from build123d import *

# Parameters (mm, degrees)
SKETCH_1_R          = 3
EXTRUDE_1_DEPTH     = 15
SKETCH_2_R          = 5
CUT_EXTRUDE_1_DEPTH = 30


with BuildPart() as part:
    # 草图1 → 凸台-拉伸1 (new, symmetric)
    with BuildSketch(Plane.XY):
        with BuildLine():
            Line((8, 0), (12, 0))
            ThreePointArc((12, 0), (17.656854249, -2.343145751), (20, -8))
            Line((20, -8), (20, -180))
            Line((20, -180), (0, -180))
            Line((0, -180), (0, -8))
            ThreePointArc((0, -8), (2.343145751, -2.343145751), (8, 0))
        make_face()
        with Locations((8, -8)):
            Circle(SKETCH_1_R, mode=Mode.SUBTRACT)
    extrude(amount=EXTRUDE_1_DEPTH, both=True)

    # 草图2 → 切除-拉伸1 (cut)
    with BuildSketch(Plane.XZ.offset(180)):
        with Locations(Location((10, 0, 0), (0, 0, 270))):
            Circle(SKETCH_2_R)
    extrude(amount=-CUT_EXTRUDE_1_DEPTH, mode=Mode.SUBTRACT)


solid = part.part
Model file for the job. Use its own axes, mm. A direction names the side the tool comes from. Round coordinates to 2 decimals unless told otherwise and drop trailing zeros. Loops run counter-clockwise (first coordinate to the right, second up) from the corner with the lowest first, then second, coordinate; pieces in that order, holes last.
1. Wall check: probe 1 along X at (y, z) = (-169.5, 0); probe 2 along Y at (x, z) = (8, -2.5); probe 3 along Y at (x, z) = (8, -4.75). Give the ranges that are in metal, low to high.
Check values:
probe 1: x = 0 to 5, 15 to 20
probe 2: y = -150 to -11, -5 to 0
probe 3: y = -180 to -11, -5 to 0
2. Tool access for faces 4 (the cylindrical face through (17.594, -2.281, 0.21)), 5 (the cylindrical face through (14.957, -165.21, 0.651)): list every direction of +Z, -Z, +X, -X, +Y, -Y with a clear straight run to the whole face (end or side of a thin tool).
Check values:
face 4: +Z, -Z, +X, +Y
face 5: -Y
3. Mould opens along X. For faces 1 (the flat face through (10, -150, 0)), 2 (the flat face through (20, -93, 0)), 3 (the flat face through (10, -89, 15)) say: +X half, -X half, draft (parallel to the pull), parting line (faces both ways), or undercut.
Check values:
face 1: undercut
face 2: +X half
face 3: draft
4. Drop flat-ended pins along their axis: P1, Ø6, axis at x = 13.5, z = 3, coming from the +Y side; P2, Ø2, axis at x = 6, z = -11, coming from the +Y side; P3, Ø3.5, axis at x = 8, y = -8, coming from the +Z side. Give the stop position or say it passes through.
Check values:
P1: stops at y = 0
P2: stops at y = -0.06
P3: passes through
5. Band-saw the part on B-B, the plane y = -158. List the corners of the cut face in (x, z).
Check values:
outline: (0, -15) - (20, -15) - (20, 15) - (0, 15) - close; hole circle Ø10 at (10, 0)
6. Band-saw the part on A-A, the plane z = 0. List the corners of the cut face in (x, y), and give its area (3 significant figures).
Check values:
outline: (0, -180) - (5, -180) - (5, -150) - (15, -150) - (15, -180) - (20, -180) - (20, -8) arc R8 ccw to (12, 0) - (8, 0) arc R8 ccw to (0, -8) - close; hole circle Ø6 at (8, -8)
area: 3,240 mm2
